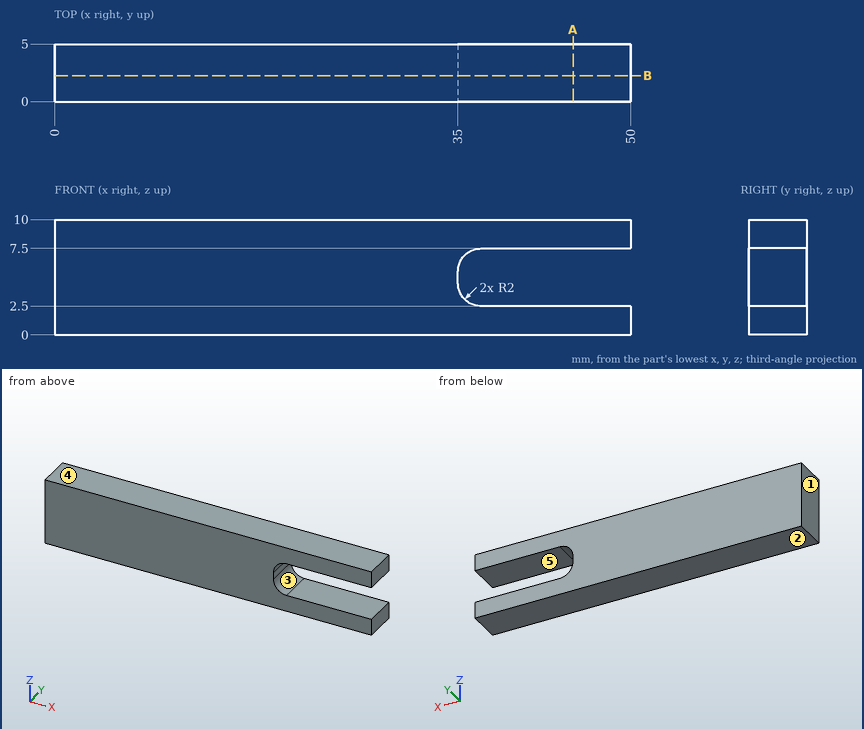
Design review of the part shown in the three views and the two pictorial views. Dimensions are in mm from the part's minimum x, y and z. A direction names the side the tool comes from. Round coordinates to 2 decimals unless told otherwise and drop trailing zeros. Write each loop counter-clockwise with the first axis right and the second up, starting at its lowest first coordinate (ties: lowest second). Pieces come first, ordered by that corner, then holes. Notation, with made-up numbers: (-2, 4.25) - (33, 4.25) arc R21 cw to (33, 8.25) - close; hole circle Ø4 at (46.5, 76.5). An arc over 180 degrees is marked (long way). Write item = value, one per line. Start each with the question number.
1. Wall thickness on L1, parallel to Z at x = 44, y = 1.45; L2, parallel to X at y = 0.3, z = 5.25; L3, parallel to X at y = 4.3, z = 7: over which ranges is each line inside the solid? List them lowest first.
2. Consider section A-A on x = 45. State the section outline as (y, z) points, plus the area to 3 significant figures.
3. For the marked faces 4 and 5, list the 3-axis set-ups (+Z, -Z, +X, -X, +Y, -Y) from which the entire face can be reached by the end or side of a thin tool; tool diameter is ignored.
4. Consider section B-B on y = 2.25. State the section outline as (x, z) points, plus the area to 3 significant figures.
5. Draft analysis for pull direction Z (two halves, no side actions). For the marked faces 1, 2 and 3, state which applies: released by +Z, released by -Z, zero draft, split by the parting line, or undercut.
6. For pin 1 Ø1 at (y, z) = (2, 8) entering from -X; pin 2 Ø1.1 at (y, z) = (3.5, 5) entering from +X, all flat-tipped, find the tip position at first contact; note any pin that passes through.
Evaluation:
q1.L1 = 0 to 2.5, 7.5 to 10
q1.L2 = 0 to 35
q1.L3 = 0 to 35.68
q2.outline = (0, 0) - (5, 0) - (5, 2.5) - (0, 2.5) - close; (0, 7.5) - (5, 7.5) - (5, 10) - (0, 10) - close
q2.area = 25.0 mm2
q3.face_4 = +Z, +X, -X, +Y, -Y
q3.face_5 = +X, +Y, -Y
q4.outline = (0, 0) - (50, 0) - (50, 2.5) - (37, 2.5) arc R2 cw to (35, 4.5) - (35, 5.5) arc R2 cw to (37, 7.5) - (50, 7.5) - (50, 10) - (0, 10) - close
q4.area = 427 mm2
q5.face_1 = zero draft
q5.face_2 = released by -Z
q5.face_3 = undercut
q6.pin_1 = 0
q6.pin_2 = 35
